Build history of the part. All positions in model axes, mm. Give positions to 0.01 mm unless a question says otherwise; leave off trailing zeros. Loops run counter-clockwise (first coordinate to the right, second up) from the corner with the lowest first, then second, coordinate; pieces in that order, holes last. Notation, with made-up numbers: (81.25, 86) -> (85.25, 86) arc R29 cw to (85.25, 106) -> close; hole circle Ø11 at (82.5, 56.5). An arc over 180 degrees is marked (long way). Answer in a Markdown table with one row per item. Add a question column.
from build123d import *

# Parameters (mm, degrees)
SKETCH_1_W          = 30
SKETCH_1_H          = 20
EXTRUDE_1_DEPTH     = 10
SKETCH_2_R          = 1.6
CUT_EXTRUDE_1_DEPTH = 38.416573868


with BuildPart() as part:
    # 草图1 → 凸台-拉伸1 (new body)
    with BuildSketch(Plane.XY):
        with Locations((15, -10)):
            Rectangle(SKETCH_1_W, SKETCH_1_H)
    extrude(amount=EXTRUDE_1_DEPTH)

    # 草图2 → 切除-拉伸1 (cut, through all)
    with BuildSketch(Plane.XY.offset(10)):
        with Locations(Location((10, -5, 0), (0, 0, 180))):
            Circle(SKETCH_2_R)
        with Locations((10, -15)):
            Circle(SKETCH_2_R)
        with Locations(Location((20, -15, 0), (0, 0, 180))):
            Circle(SKETCH_2_R)
        with Locations((20, -5)):
            Circle(SKETCH_2_R)
    extrude(amount=-CUT_EXTRUDE_1_DEPTH, mode=Mode.SUBTRACT)


solid = part.part
(1) Saw through at C-C, the plane y = -15. List the corners of the cut face in (x, z), then the cut area to 3 significant figures.
(2) Wall check: line 1 along Y through (x, z) = (10, 6); line 2 along Y through (x, z) = (11, 2.5); line 3 along X through (y, z) = (-6, 6.5). Give the ranges that are in metal, low to high. Write a range as from..to.
(3) Saw through at A-A, the plane x = 20. List the corners of the cut face in (y, z), then the cut area to 3 significant figures.
(4) Two-plate mould, pull along X, no slides. Class faces 1 (the flat face through (15, 0, 5)), 2 (the flat face through (0, -10, 5)), 3 (the cylindrical face through (18.82, -3.92, 5.07)), 4 (the cylindrical face through (21.18, -16.08, 5.07)): released by +X, released by -X, zero draft, split by the parting line, or undercut.
(5) Saw through at B-B, the plane z = 3. List the corners of the cut face in (x, y).
Worked answers:
| question | item | result |
|---|---|---|
| 1 | outline | (0, 0) -> (8.4, 0) -> (8.4, 10) -> (0, 10) -> close; (11.6, 0) -> (18.4, 0) -> (18.4, 10) -> (11.6, 10) -> close; (21.6, 0) -> (30, 0) -> (30, 10) -> (21.6, 10) -> close |
| 1 | area | 236 mm^2 |
| 2 | line 1 | -20..-16.6, -13.4..-6.6, -3.4..0 |
| 2 | line 2 | -20..-16.25, -13.75..-6.25, -3.75..0 |
| 2 | line 3 | 0..8.75, 11.25..18.75, 21.25..30 |
| 3 | outline | (-20, 0) -> (-16.6, 0) -> (-16.6, 10) -> (-20, 10) -> close; (-13.4, 0) -> (-6.6, 0) -> (-6.6, 10) -> (-13.4, 10) -> close; (-3.4, 0) -> (0, 0) -> (0, 10) -> (-3.4, 10) -> close |
| 3 | area | 136 mm^2 |
| 4 | face 1 | zero draft |
| 4 | face 2 | released by -X |
| 4 | face 3 | undercut |
| 4 | face 4 | undercut |
| 5 | outline | (0, -20) -> (30, -20) -> (30, 0) -> (0, 0) -> close; hole circle Ø3.2 at (10, -15); hole circle Ø3.2 at (10, -5); hole circle Ø3.2 at (20, -15); hole circle Ø3.2 at (20, -5) |
